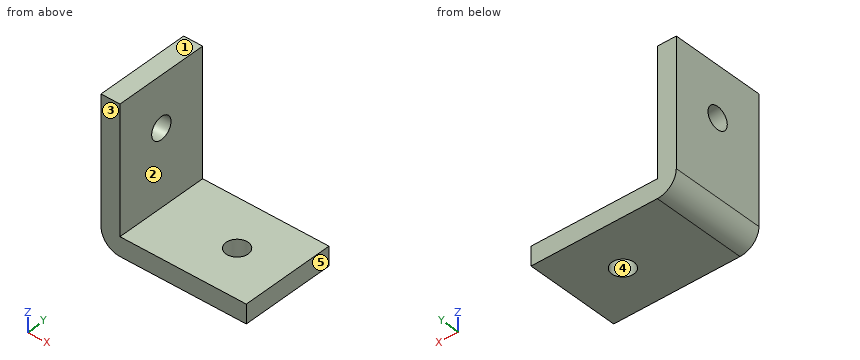
from build123d import *

# Parameters (mm, degrees)
SKETCH1_W           = 23
SKETCH1_H           = 15
BOSS_EXTRUDE1_DEPTH = 3
SKETCH10_W          = 3
SKETCH10_H          = 15
BOSS_EXTRUDE2_DEPTH = 20
SKETCH13_R          = 1.75
CUT_EXTRUDE3_DEPTH  = 24
SKETCH14_R          = 1.75
CUT_EXTRUDE4_DEPTH  = 24
FILLET1_R           = 3


with BuildPart() as part:
    # Sketch1 → Boss-Extrude1 (new body)
    with BuildSketch(Plane.XY):
        Rectangle(SKETCH1_W, SKETCH1_H)
    extrude(amount=BOSS_EXTRUDE1_DEPTH)

    # Sketch10 → Boss-Extrude2 (add)
    with BuildSketch(Plane.XY.offset(3)):
        with Locations((-10, 0)):
            Rectangle(SKETCH10_W, SKETCH10_H)
    extrude(amount=BOSS_EXTRUDE2_DEPTH)

    # Sketch13 → Cut-Extrude3 (cut, through all)
    with BuildSketch(Plane(origin=(0, 0, 0), x_dir=(-1, 0, 0), z_dir=(0, 0, -1))):
        with Locations((-3.5, 0)):
            Circle(SKETCH13_R)
    extrude(amount=-CUT_EXTRUDE3_DEPTH, mode=Mode.SUBTRACT)

    # Sketch14 → Cut-Extrude4 (cut, through all)
    with BuildSketch(Plane.ZY.offset(11.5)):
        with Locations((15, 0)):
            Circle(SKETCH14_R)
    extrude(amount=-CUT_EXTRUDE4_DEPTH, mode=Mode.SUBTRACT)

    # Fillet1
    fillet1_edges = [part.edges().sort_by_distance(p)[0] for p in [
        (-11.5, 0, 0),
    ]]
    fillet(fillet1_edges, radius=FILLET1_R)


solid = part.part
For this review, take the finished solid that the model builds, in its own axes (mm). Face numbers are marked on the shaded views. A direction names the side the tool comes from. Coordinates: 2 decimals unless noted, no trailing zeros. Loops run counter-clockwise (first coordinate to the right, second up) from the corner with the lowest first, then second, coordinate; pieces in that order, holes last. Notation, with made-up numbers: (6, 33.5) - (23, 33.5) arc R30 cw to (23, 62.5) - close; hole circle Ø9 at (60, 27). An arc over 180 degrees is marked (long way). Use a Markdown table: item, result. Add a question column.
Item 1: Insertion check: pin 1 Ø12 at (x, z) = (4.5, 6.5) entering from +Y; pin 2 Ø7.5 at (y, z) = (3, 8.5) entering from +X; pin 3 Ø3 at (x, y) = (3.5, 0) entering from +Z. Each pin has a flat end and moves straight along its axis. Give the tip position at first contact, or say it passes through.
Item 2: Mouldability with a two-part tool opening along Y and no side actions: class the marked faces 3, 4 and 5 as pulls with the +Y half, pulls with the -Y half, needs draft (parallel to the pull), parting line crosses it, or undercut.
Item 3: We need section A-A (y = 0). Give the boundary of the cut face in (x, z), and give its area (3 significant figures).
Item 4: For line 1 (Y direction, x = 3.5, z = 1.5); line 2 (Z direction, x = 6.5, y = 0.25); line 3 (X direction, y = -1.5, z = 1.75), list the stretches that pass through material, from the lowest coordinate up.
Item 5: We need section B-B (z = 15). Give the boundary of the cut face in (x, y).
Item 6: We need section C-C (x = 3.5). Give the boundary of the cut face in (y, z).
Item 7: We need section D-D (y = 2.5). Give the boundary of the cut face in (x, z).
Item 8: Tool access review of the marked faces 1 and 2: name each direction out of +Z, -Z, +X, -X, +Y, -Y from which nothing blocks a thin tool from reaching the whole face with its end or side.
Results list:
| question | item | result |
|---|---|---|
| 1 | pin 1 | stops at y = 7.5 |
| 1 | pin 2 | stops at x = -8.5 |
| 1 | pin 3 | passes through |
| 2 | face 3 | pulls with the -Y half |
| 2 | face 4 | undercut |
| 2 | face 5 | needs draft |
| 3 | outline | (-11.5, 3) arc R3 ccw to (-8.5, 0) - (1.75, 0) - (1.75, 3) - (-8.5, 3) - (-8.5, 13.25) - (-11.5, 13.25) - close; (-11.5, 16.75) - (-8.5, 16.75) - (-8.5, 23) - (-11.5, 23) - close; (5.25, 0) - (11.5, 0) - (11.5, 3) - (5.25, 3) - close |
| 3 | area | 106 mm^2 |
| 4 | line 1 | y = -7.5 to -1.75, 1.75 to 7.5 |
| 4 | line 2 | z = 0 to 3 |
| 4 | line 3 | x = -11.23 to 2.6, 4.4 to 11.5 |
| 5 | outline | (-11.5, -7.5) - (-8.5, -7.5) - (-8.5, -1.75) - (-11.5, -1.75) - close; (-11.5, 1.75) - (-8.5, 1.75) - (-8.5, 7.5) - (-11.5, 7.5) - close |
| 6 | outline | (-7.5, 0) - (-1.75, 0) - (-1.75, 3) - (-7.5, 3) - close; (1.75, 0) - (7.5, 0) - (7.5, 3) - (1.75, 3) - close |
| 7 | outline | (-11.5, 3) arc R3 ccw to (-8.5, 0) - (11.5, 0) - (11.5, 3) - (-8.5, 3) - (-8.5, 23) - (-11.5, 23) - close |
| 8 | face 1 | +Z, +X, -X, +Y, -Y |
| 8 | face 2 | +Z, +X, +Y, -Y |
